from build123d import *

# Parameters (mm, degrees)
SALIENTE_EXTRUIR1_DEPTH                              = 35
SALIENTE_EXTRUIR2_DEPTH                              = 5
CORTAR_EXTRUIR1_DEPTH                                = 5
CROQUIS4_R                                           = 9.25
CORTAR_EXTRUIR2_DEPTH                                = 5
REFRENTADO_PARA_TORNILLO_TAP_N_CON_CABEZ_D           = 4.5
REFRENTADO_PARA_TORNILLO_TAP_N_CON_CABEZ_CSINK_D     = 8.96
REFRENTADO_PARA_TORNILLO_TAP_N_CON_CABEZ_CSINK_ANGLE = 90
CROQUIS7_R                                           = 2
CROQUIS7_R_2                                         = 0.9
SALIENTE_EXTRUIR3_DEPTH                              = 5
CROQUIS8_R                                           = 1.5
CROQUIS8_R_2                                         = 0.9
SALIENTE_EXTRUIR4_DEPTH                              = 1
CROQUIS9_R                                           = 1.5
SALIENTE_EXTRUIR5_DEPTH                              = 5
SALIENTE_EXTRUIR6_REACH                              = 91.967
CROQUIS10_R                                          = 4
CROQUIS10_R_2                                        = 0.9
CORTAR_EXTRUIR3_REACH                                = 91.967
CROQUIS10_2_R                                        = 0.9


with BuildPart() as part:
    # Croquis2 → Saliente-Extruir1 (new body)
    with BuildSketch(Plane(origin=(0, 0, 0), x_dir=(1, 0, 0), z_dir=(0, 1, 0))):
        with BuildLine():
            Line((62, 3), (62, 35))
            Line((62, 35), (62, 40))
            ThreePointArc((62, 40), (57.606601718, 50.606601718), (47, 55))
            Line((47, 55), (3, 55))
            ThreePointArc((3, 55), (-7.606601718, 50.606601718), (-12, 40))
            Line((-12, 40), (-12, 35))
            Line((-12, 35), (-12, 3))
            ThreePointArc((-12, 3), (-7.606601718, -7.606601718), (3, -12))
            Line((3, -12), (47, -12))
            ThreePointArc((47, -12), (57.606601718, -7.606601718), (62, 3))
        make_face()
        with BuildLine():
            Line((58, 3), (58, 35))
            ThreePointArc((58, 35), (54.778174593, 42.778174593), (47, 46))
            Line((47, 46), (3, 46))
            ThreePointArc((3, 46), (-4.778174593, 42.778174593), (-8, 35))
            Line((-8, 35), (-8, 3))
            ThreePointArc((-8, 3), (-4.778174593, -4.778174593), (3, -8))
            Line((3, -8), (47, -8))
            ThreePointArc((47, -8), (54.778174593, -4.778174593), (58, 3))
        make_face(mode=Mode.SUBTRACT)
    extrude(amount=SALIENTE_EXTRUIR1_DEPTH)

    # Croquis2<2> → Saliente-Extruir2 (add)
    with BuildSketch(Plane(origin=(0, 0, 0), x_dir=(1, 0, 0), z_dir=(0, 1, 0))):
        with BuildLine():
            Line((47, 46), (3, 46))
            ThreePointArc((3, 46), (-4.778174593, 42.778174593), (-8, 35))
            Line((-8, 35), (-8, 3))
            ThreePointArc((-8, 3), (-4.778174593, -4.778174593), (3, -8))
            Line((3, -8), (47, -8))
            ThreePointArc((47, -8), (54.778174593, -4.778174593), (58, 3))
            Line((58, 3), (58, 35))
            ThreePointArc((58, 35), (54.778174593, 42.778174593), (47, 46))
        make_face()
    extrude(amount=SALIENTE_EXTRUIR2_DEPTH)

    # Croquis3 → Cortar-Extruir1 (cut)
    with BuildSketch(Plane.XY.offset(-46)):
        Polygon((39.145081595, 20), (32.072540798, 32.25), (17.927459202, 32.25), (10.854918405, 20), (17.927459202, 7.75), (32.072540798, 7.75), align=None)
    extrude(amount=-CORTAR_EXTRUIR1_DEPTH, mode=Mode.SUBTRACT)

    # Croquis4 → Cortar-Extruir2 (cut)
    with BuildSketch(Plane.XY.offset(-51)):
        with Locations((25, 20)):
            Circle(CROQUIS4_R)
    extrude(amount=-CORTAR_EXTRUIR2_DEPTH, mode=Mode.SUBTRACT)

    # Refrentado para tornillo tapón con cabeza plana de clavija de M41 (through all)
    with Locations(Plane(origin=(0, 5, 0), x_dir=(1, 0, 0), z_dir=(0, 1, 0))):
        with Locations((0, 19), (50, 19), (25, 0), (25, 38)):
            CounterSinkHole(REFRENTADO_PARA_TORNILLO_TAP_N_CON_CABEZ_D / 2, REFRENTADO_PARA_TORNILLO_TAP_N_CON_CABEZ_CSINK_D / 2, counter_sink_angle=REFRENTADO_PARA_TORNILLO_TAP_N_CON_CABEZ_CSINK_ANGLE)

    # Croquis7 → Saliente-Extruir3 (add)
    # profile 1 of 3: a face of its own
    with BuildSketch(Plane(origin=(0, 5, 0), x_dir=(1, 0, 0), z_dir=(0, 1, 0))):
        with Locations(Location((3, 3, 0), (0, 0, 270))):
            Circle(CROQUIS7_R)
        with Locations(Location((3, 3, 0), (0, 0, 270))):
            Circle(CROQUIS7_R_2, mode=Mode.SUBTRACT)
    # profile 2 of 3: a face of its own
    with BuildSketch(Plane(origin=(0, 5, 0), x_dir=(1, 0, 0), z_dir=(0, 1, 0))):
        with Locations(Location((47, 3, 0), (0, 0, 270))):
            Circle(CROQUIS7_R)
        with Locations(Location((47, 3, 0), (0, 0, 270))):
            Circle(CROQUIS7_R_2, mode=Mode.SUBTRACT)
    # profile 3 of 3: a face of its own
    with BuildSketch(Plane(origin=(0, 5, 0), x_dir=(1, 0, 0), z_dir=(0, 1, 0))):
        with Locations(Location((47, 35, 0), (0, 0, 270))):
            Circle(CROQUIS7_R)
        with Locations(Location((47, 35, 0), (0, 0, 270))):
            Circle(CROQUIS7_R_2, mode=Mode.SUBTRACT)
    extrude(amount=SALIENTE_EXTRUIR3_DEPTH)

    # Croquis8 → Saliente-Extruir4 (add)
    # profile 1 of 3: a face of its own
    with BuildSketch(Plane(origin=(0, 10, 0), x_dir=(1, 0, 0), z_dir=(0, 1, 0))):
        with Locations(Location((47, 35, 0), (0, 0, 270))):
            Circle(CROQUIS8_R)
        with Locations(Location((47, 35, 0), (0, 0, 270))):
            Circle(CROQUIS8_R_2, mode=Mode.SUBTRACT)
    # profile 2 of 3: a face of its own
    with BuildSketch(Plane(origin=(0, 10, 0), x_dir=(1, 0, 0), z_dir=(0, 1, 0))):
        with Locations(Location((47, 3, 0), (0, 0, 270))):
            Circle(CROQUIS8_R)
        with Locations(Location((47, 3, 0), (0, 0, 270))):
            Circle(CROQUIS8_R_2, mode=Mode.SUBTRACT)
    # profile 3 of 3: a face of its own
    with BuildSketch(Plane(origin=(0, 10, 0), x_dir=(1, 0, 0), z_dir=(0, 1, 0))):
        with Locations(Location((3, 3, 0), (0, 0, 270))):
            Circle(CROQUIS8_R)
        with Locations(Location((3, 3, 0), (0, 0, 270))):
            Circle(CROQUIS8_R_2, mode=Mode.SUBTRACT)
    extrude(amount=SALIENTE_EXTRUIR4_DEPTH)

    # Croquis9 → Saliente-Extruir5 (add)
    with BuildSketch(Plane(origin=(0, 5, 0), x_dir=(1, 0, 0), z_dir=(0, 1, 0))):
        with Locations(Location((3, 35, 0), (0, 0, 270))):
            Circle(CROQUIS9_R)
    extrude(amount=SALIENTE_EXTRUIR5_DEPTH)

    # Croquis10 → Saliente-Extruir6 (add, up to next)
    with BuildSketch(Plane(origin=(0, 35, 0), x_dir=(1, 0, 0), z_dir=(0, 1, 0)), mode=Mode.PRIVATE) as saliente_extruir6_sk1:
        with Locations((-4.778174593, -4.778174593)):
            Circle(CROQUIS10_R)
        with Locations((-4.778174593, -4.778174593)):
            Circle(CROQUIS10_R_2, mode=Mode.SUBTRACT)
    saliente_extruir6_tool1 = extrude(saliente_extruir6_sk1.sketch, amount=-SALIENTE_EXTRUIR6_REACH, mode=Mode.PRIVATE) - part.part
    # Croquis10 → Saliente-Extruir6 (add, up to next)
    with BuildSketch(Plane(origin=(0, 35, 0), x_dir=(1, 0, 0), z_dir=(0, 1, 0)), mode=Mode.PRIVATE) as saliente_extruir6_sk2:
        with Locations((-4.778174593, 42.778174593)):
            Circle(CROQUIS10_R)
        with Locations((-4.778174593, 42.778174593)):
            Circle(CROQUIS10_R_2, mode=Mode.SUBTRACT)
    saliente_extruir6_tool2 = extrude(saliente_extruir6_sk2.sketch, amount=-SALIENTE_EXTRUIR6_REACH, mode=Mode.PRIVATE) - part.part
    # Croquis10 → Saliente-Extruir6 (add, up to next)
    with BuildSketch(Plane(origin=(0, 35, 0), x_dir=(1, 0, 0), z_dir=(0, 1, 0)), mode=Mode.PRIVATE) as saliente_extruir6_sk3:
        with Locations((54.778174593, 42.778174593)):
            Circle(CROQUIS10_R)
        with Locations((54.778174593, 42.778174593)):
            Circle(CROQUIS10_R_2, mode=Mode.SUBTRACT)
    saliente_extruir6_tool3 = extrude(saliente_extruir6_sk3.sketch, amount=-SALIENTE_EXTRUIR6_REACH, mode=Mode.PRIVATE) - part.part
    # Croquis10 → Saliente-Extruir6 (add, up to next)
    with BuildSketch(Plane(origin=(0, 35, 0), x_dir=(1, 0, 0), z_dir=(0, 1, 0)), mode=Mode.PRIVATE) as saliente_extruir6_sk4:
        with Locations((54.778174593, -4.778174593)):
            Circle(CROQUIS10_R)
        with Locations((54.778174593, -4.778174593)):
            Circle(CROQUIS10_R_2, mode=Mode.SUBTRACT)
    saliente_extruir6_tool4 = extrude(saliente_extruir6_sk4.sketch, amount=-SALIENTE_EXTRUIR6_REACH, mode=Mode.PRIVATE) - part.part
    add(saliente_extruir6_tool1.solids().sort_by_distance((-8.665038, 35, 4.778175))[0])
    add(saliente_extruir6_tool2.solids().sort_by_distance((-8.665038, 35, -42.778175))[0])
    add(saliente_extruir6_tool3.solids().sort_by_distance((50.891312, 35, -42.778175))[0])
    add(saliente_extruir6_tool4.solids().sort_by_distance((50.891312, 35, 4.778175))[0])

    # Croquis10<2> → Cortar-Extruir3 (cut, up to next)
    with BuildSketch(Plane(origin=(0, 35, 0), x_dir=(1, 0, 0), z_dir=(0, 1, 0)), mode=Mode.PRIVATE) as cortar_extruir3_sk1:
        with Locations(Location((-4.778174593, -4.778174593, 0), (0, 0, 270))):
            Circle(CROQUIS10_2_R)
    cortar_extruir3_tool1 = extrude(cortar_extruir3_sk1.sketch, amount=-CORTAR_EXTRUIR3_REACH, mode=Mode.PRIVATE) & part.part
    # Croquis10<2> → Cortar-Extruir3 (cut, up to next)
    with BuildSketch(Plane(origin=(0, 35, 0), x_dir=(1, 0, 0), z_dir=(0, 1, 0)), mode=Mode.PRIVATE) as cortar_extruir3_sk2:
        with Locations(Location((54.778174593, -4.778174593, 0), (0, 0, 270))):
            Circle(CROQUIS10_2_R)
    cortar_extruir3_tool2 = extrude(cortar_extruir3_sk2.sketch, amount=-CORTAR_EXTRUIR3_REACH, mode=Mode.PRIVATE) & part.part
    # Croquis10<2> → Cortar-Extruir3 (cut, up to next)
    with BuildSketch(Plane(origin=(0, 35, 0), x_dir=(1, 0, 0), z_dir=(0, 1, 0)), mode=Mode.PRIVATE) as cortar_extruir3_sk3:
        with Locations(Location((-4.778174593, 42.778174593, 0), (0, 0, 270))):
            Circle(CROQUIS10_2_R)
    cortar_extruir3_tool3 = extrude(cortar_extruir3_sk3.sketch, amount=-CORTAR_EXTRUIR3_REACH, mode=Mode.PRIVATE) & part.part
    # Croquis10<2> → Cortar-Extruir3 (cut, up to next)
    with BuildSketch(Plane(origin=(0, 35, 0), x_dir=(1, 0, 0), z_dir=(0, 1, 0)), mode=Mode.PRIVATE) as cortar_extruir3_sk4:
        with Locations(Location((54.778174593, 42.778174593, 0), (0, 0, 270))):
            Circle(CROQUIS10_2_R)
    cortar_extruir3_tool4 = extrude(cortar_extruir3_sk4.sketch, amount=-CORTAR_EXTRUIR3_REACH, mode=Mode.PRIVATE) & part.part
    add(cortar_extruir3_tool1.solids().sort_by_distance((-4.778175, 35, 4.778175))[0], mode=Mode.SUBTRACT)
    add(cortar_extruir3_tool2.solids().sort_by_distance((54.778175, 35, 4.778175))[0], mode=Mode.SUBTRACT)
    add(cortar_extruir3_tool3.solids().sort_by_distance((-4.778175, 35, -42.778175))[0], mode=Mode.SUBTRACT)
    add(cortar_extruir3_tool4.solids().sort_by_distance((54.778175, 35, -42.778175))[0], mode=Mode.SUBTRACT)


solid = part.part
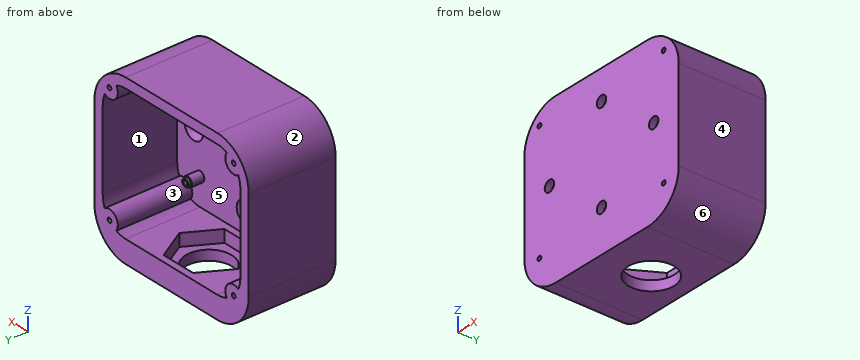
For this review, take the finished solid that the model builds, in its own axes (mm). Face numbers are marked on the shaded views. A direction names the side the tool comes from. Round coordinates to 2 decimals unless told otherwise and drop trailing zeros. Write each loop counter-clockwise with the first axis right and the second up, starting at its lowest first coordinate (ties: lowest second). Pieces come first, ordered by that corner, then holes. Notation, with made-up numbers: (28, 64) -> (62, 64) arc R26 cw to (62, 85) -> close; hole circle Ø5 at (88, -17). An arc over 180 degrees is marked (long way). Put each result on its own line as item: value.
Q1. Consider section A-A on z = -19. State the section outline as (x, y) points.
Determined:
outline: (-12, 0) -> (-2.25, 0) -> (-2.25, 2.77) -> (-4.48, 5) -> (-8, 5) -> (-8, 35) -> (-12, 35) -> close; (2.25, 0) -> (47.75, 0) -> (47.75, 2.77) -> (45.52, 5) -> (4.48, 5) -> (2.25, 2.77) -> close; (52.25, 0) -> (62, 0) -> (62, 35) -> (58, 35) -> (58, 5) -> (54.48, 5) -> (52.25, 2.77) -> close
Q2. Consider section C-C on x = 12.5. State the section outline as (y, z) points.
Determined:
outline: (0, -55) -> (35, -55) -> (35, -46) -> (22.85, -46) -> (22.85, -51) -> (17.15, -51) -> (17.15, -46) -> (5, -46) -> (5, 8) -> (35, 8) -> (35, 12) -> (0, 12) -> close
Q3. Machinability: for the marked faces 5 and 6, which of the approach directions +Z, -Z, +X, -X, +Y, -Y give a long, thin tool a straight path to every point of the face, cutting with its end or side? Answer none if there is none.
Determined:
face 5: +Y
face 6: -Z, +X, +Y, -Y
Q4. Clearance check with flat-ended pins moving along their axes: pin 1 Ø6 at (x, z) = (25, -38) entering from +Y; pin 2 Ø2 at (x, z) = (47, -35) entering from +Y; pin 3 Ø5 at (x, y) = (51, 31.5) entering from +Z. State where each tip first meets the part, or that it passes through.
Determined:
pin 1: stops at y = 3.52
pin 2: stops at y = 11
pin 3: stops at z = 11.92
Q5. The part is to be moulded in two halves that separate along X. For the marked faces 1, 2, 3 and 4, say which applies: released by +X, released by -X, zero draft, split by the parting line, or undercut.
Determined:
face 1: undercut
face 2: released by -X
face 3: undercut
face 4: released by +X
Q6. Consider section B-B on y = 4. Give the number of separate pieces and of enclosed holes in the cut face, and give its area (3 significant figures).
Determined:
separate pieces: 1
enclosed holes: 8
area: 4,600 mm^2
Q7. To check wall thickness, follow L1, parallel to X at y = 24.5, z = -10.5; L2, parallel to Z at x = 25, y = 1; L3, parallel to X at y = 1.55, z = -38. State the ranges of each line that lie inside material, in increasing order. Write a range as [from, to].
Determined:
L1: x = [-12, -8], [58, 62]
L2: z = [-55, -40.25], [-35.75, -2.25], [2.25, 12]
L3: x = [-12, 22.75], [27.25, 62]
